Geometry: see drawing. Coordinates: mm, zero at the bounding-box minimum. Coordinates: 2 decimals unless noted, no trailing zeros. Loops run counter-clockwise (first coordinate to the right, second up) from the corner with the lowest first, then second, coordinate; pieces in that order, holes last.
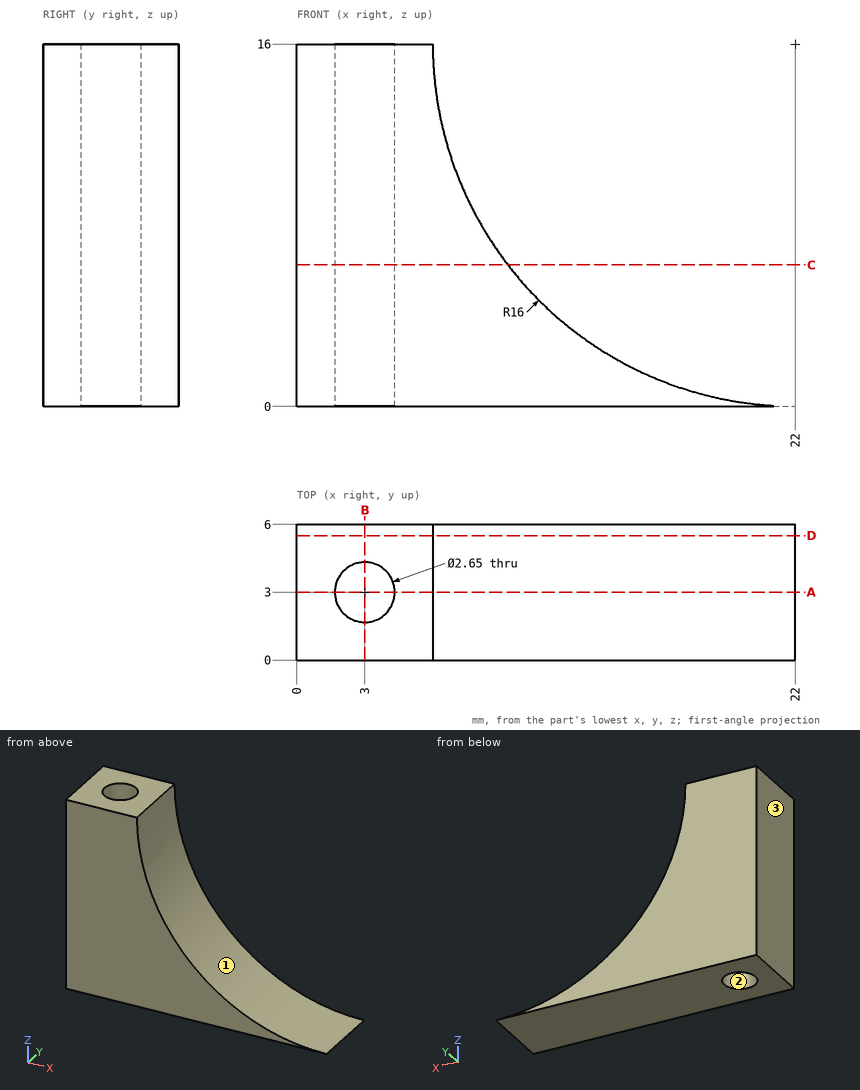
Item 1: Line query: L1, parallel to Y at x = 3, z = 9 (3 decimals); L2, parallel to X at y = 2.2, z = 15; L3, parallel to Y at x = 3.5, z = 9.25. Output: solid intervals per line, ascending.
Result:
L1: y = 0 to 1.675, 4.325 to 6
L2: x = 0 to 1.94, 4.06 to 6.03
L3: y = 0 to 1.77, 4.23 to 6
Item 2: Section query C-C (z = 6.25). Output: boundary loops of the cut face in (x, y) (3 decimals).
Result:
outline: (0, 0) - (9.314, 0) - (9.314, 6) - (0, 6) - close; hole circle Ø2.65 at (3, 3)
Item 3: Section query A-A (y = 3). Output: boundary loops of the cut face in (x, z) (3 decimals), then the cut area to 3 significant figures.
Result:
outline: (0, 0) - (1.675, 0) - (1.675, 16) - (0, 16) - close; (4.325, 0) - (22, 0) arc R16 cw to (6, 16) - (4.325, 16) - close
area: 109 mm2
Item 4: Section query B-B (x = 3). Output: boundary loops of the cut face in (y, z) (3 decimals).
Result:
outline: (0, 0) - (1.675, 0) - (1.675, 16) - (0, 16) - close; (4.325, 0) - (6, 0) - (6, 16) - (4.325, 16) - close
Item 5: Mould query, pull axis X, two halves, no side actions, for the marked faces 1, 2 and 3. Classes: +X half, -X half, draft (parallel to the pull), parting line (faces both ways), or undercut.
Result:
face 1: +X half
face 2: undercut
face 3: -X half
Item 6: Section query D-D (y = 5.5). Output: boundary loops of the cut face in (x, z), then the cut area to 3 significant figures.
Result:
outline: (0, 0) - (22, 0) arc R16 cw to (6, 16) - (0, 16) - close
area: 151 mm2
